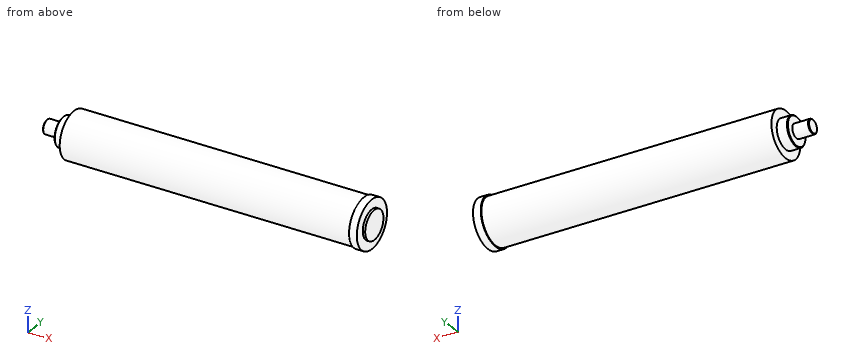
from build123d import *

# Parameters (mm, degrees)
CHANFREIN1_SIZE = 1


with BuildPart() as part:
    # Esquisse1 → Révolution1 (revolve)
    with BuildSketch(Plane.XY):
        Polygon((0, 0), (0, 11.395), (26.75, 11.395), (26.75, 23.8), (44.5, 23.8), (44.5, 37.65), (519.3, 37.65), (519.3, 39.35), (532, 39.35), (532, 23.8), (535.96, 23.8), (535.96, 0), align=None)
    revolve(axis=Axis((0, 0, 0), (1, 0, 0)))

    # Chanfrein1
    chanfrein1_edges = [part.edges().sort_by_distance(p)[0] for p in [
        (26.75, -23.8, 0),
        (0, -11.395, 0),
    ]]
    chamfer(chanfrein1_edges, length=CHANFREIN1_SIZE)


solid = part.part
Work out the finished part from the listing and answer in its coordinate system (mm). Give positions to 0.01 mm unless a question says otherwise; leave off trailing zeros. Loops run counter-clockwise (first coordinate to the right, second up) from the corner with the lowest first, then second, coordinate; pieces in that order, holes last. Notation, with made-up numbers: (8.5, 8) -> (67.5, 8) arc R24 ccw to (67.5, 38) -> close; hole circle Ø11 at (-29, -34). An arc over 180 degrees is marked (long way). Use a Markdown table: item, result. Add a question column.
1. Section C-C on x = 34.5 is taken. Determine the outline of the cut face in (y, z), and give its area (3 significant figures).
2. Flat-ended cylindrical pins translate along their axes: pin 1 Ø6 at (x, y) = (379, -3) entering from +Z; pin 2 Ø4 at (x, z) = (159, 29) entering from -Y; pin 3 Ø1 at (x, y) = (251, 27.5) entering from +Z. Find the tip coordinate at first contact, or state that the pin passes through.
3. Section D-D on z = -30.5 is taken. Determine the outline of the cut face in (x, y), and give its area (3 significant figures).
4. Find the intervals of material crossed by probe 1 along X at (y, z) = (-15.5, 21.5); probe 2 along X at (y, z) = (13, 7.5); probe 3 along Y at (x, z) = (440.5, -2.5), in increasing order.
5. Section A-A on y = 0 is taken. Determine the outline of the cut face in (x, z) (3 decimals).
Results below:
| question | item | result |
|---|---|---|
| 1 | outline | circle Ø47.6 at (0, 0) |
| 1 | area | 1,780 mm^2 |
| 2 | pin 1 | stops at z = 37.65 |
| 2 | pin 2 | stops at y = -26.24 |
| 2 | pin 3 | stops at z = 26.24 |
| 3 | outline | (44.5, -22.07) -> (519.3, -22.07) -> (519.3, -24.86) -> (532, -24.86) -> (532, 24.86) -> (519.3, 24.86) -> (519.3, 22.07) -> (44.5, 22.07) -> close |
| 3 | area | 21,600 mm^2 |
| 4 | probe 1 | x = 44.5 to 532 |
| 4 | probe 2 | x = 26.75 to 535.96 |
| 4 | probe 3 | y = -37.57 to 37.57 |
| 5 | outline | (0, -10.395) -> (1, -11.395) -> (26.75, -11.395) -> (26.75, -22.8) -> (27.75, -23.8) -> (44.5, -23.8) -> (44.5, -37.65) -> (519.3, -37.65) -> (519.3, -39.35) -> (532, -39.35) -> (532, -23.8) -> (535.96, -23.8) -> (535.96, 23.8) -> (532, 23.8) -> (532, 39.35) -> (519.3, 39.35) -> (519.3, 37.65) -> (44.5, 37.65) -> (44.5, 23.8) -> (27.75, 23.8) -> (26.75, 22.8) -> (26.75, 11.395) -> (1, 11.395) -> (0, 10.395) -> close |
